Answer from the drawing. Dimensions are ordinates in mm from the lowest x, y and z of the part. Round coordinates to 2 decimals unless told otherwise and drop trailing zeros. Write each loop counter-clockwise with the first axis right and the second up, starting at its lowest first coordinate (ties: lowest second). Pieces come first, ordered by that corner, then holes. Notation, with made-up numbers: (-14, 39) - (13, 39) arc R18 ccw to (13, 72) - close; hole circle Ø6 at (25, 40.5). An arc over 180 degrees is marked (long way). Use a Markdown table: item, result. Add a question column.
1) A cutting plane is placed at B-B (x = 30.48). Give the vertices of the cut face in (y, z).
2) This flat-tipped pin is pushed along its axis until it touches: P1, Ø6, axis at x = 119.77, z = 12.7, coming from the -Y side. Where does it stop, or does it pass through?
3) Find the intervals of material crossed by probe 1 along Z at (x, y) = (120, 1); probe 2 along X at (y, z) = (2, 9.25); probe 3 along Z at (x, y) = (28.5, 0.75) (1 decimal), in increasing order. Write a range as from..to.
4) A cutting plane is placed at A-A (z = 12.7). State how many separate pieces and enclosed holes the cut face has.
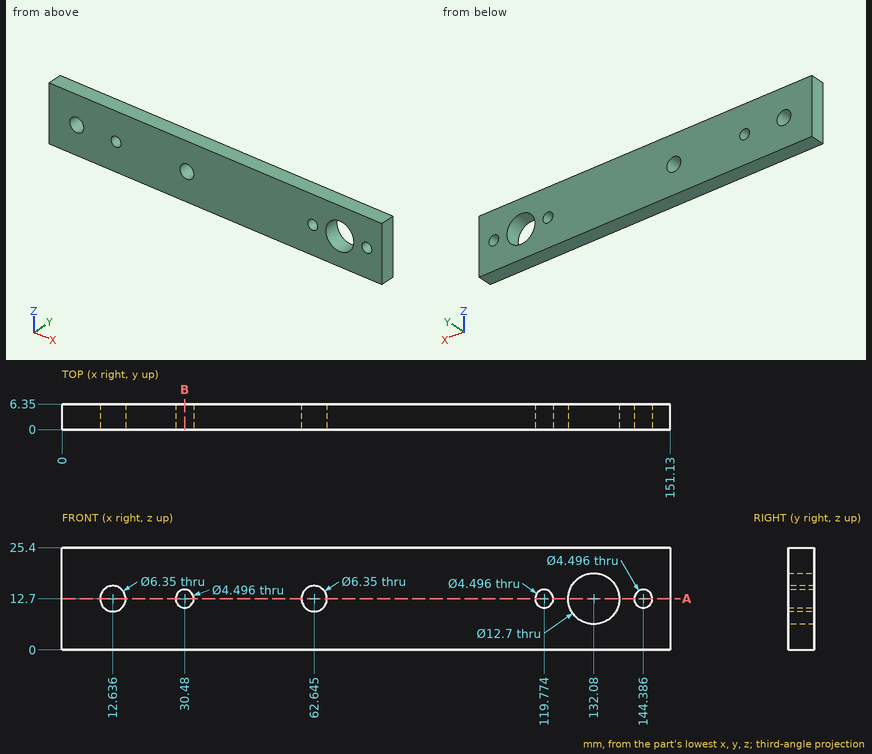
Entries:
| question | item | result |
|---|---|---|
| 1 | outline | (0, 0) - (6.35, 0) - (6.35, 10.45) - (0, 10.45) - close; (0, 14.95) - (6.35, 14.95) - (6.35, 25.4) - (0, 25.4) - close |
| 2 | P1 | stops at y = 0 |
| 3 | probe 1 | z = 0..10.46, 14.94..25.4 |
| 3 | probe 2 | x = 0..126.75, 137.41..151.13 |
| 3 | probe 3 | z = 0..11.6, 13.8..25.4 |
| 4 | separate pieces | 7 |
| 4 | enclosed holes | 0 |
